Input: part model. Units: mm. Frame: model coordinates. Face numbers are marked on the shaded views. Give positions to 0.01 mm unless a question says otherwise; leave off trailing zeros. Order: outer loops, then holes, each group sorted by start corner. A loop starts at its lowest first (then second) coordinate and runs counter-clockwise, first axis right, second up.
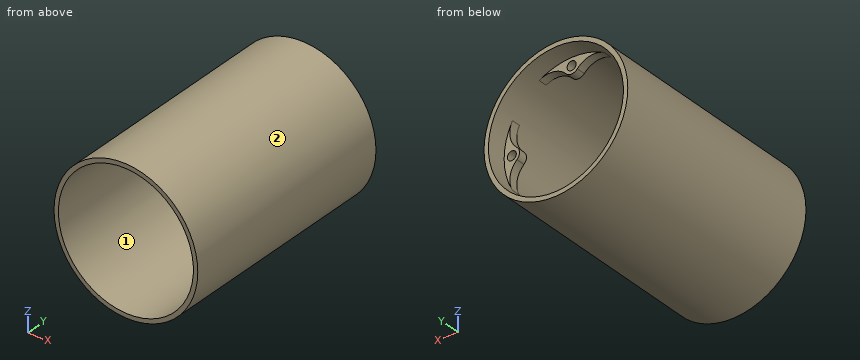
```python
from build123d import *

# Parameters (mm, degrees)
SKETCH1_R           = 32.75
SKETCH1_R_2         = 30.75
BOSS_EXTRUDE1_DEPTH = 102
SKETCH3_R           = 2.05
BOSS_EXTRUDE2_DEPTH = 4
FILLET1_R           = 10


with BuildPart() as part:
    # Sketch1 → Boss-Extrude1 (new body)
    with BuildSketch(Plane(origin=(0, 0, 0), x_dir=(1, 0, 0), z_dir=(0, 1, 0))):
        with Locations(Location((0, 0, 0), (0, 0, 270))):
            Circle(SKETCH1_R)
        with Locations(Location((0, 0, 0), (0, 0, 270))):
            Circle(SKETCH1_R_2, mode=Mode.SUBTRACT)
    extrude(amount=BOSS_EXTRUDE1_DEPTH)

    # Sketch3 → Boss-Extrude2 (add)
    # profile 1 of 4: a face of its own
    with BuildSketch(Plane(origin=(0, 93, 0), x_dir=(1, 0, 0), z_dir=(0, 1, 0))):
        with BuildLine():
            Line((-3.5, 27.25), (-3.5, 30.801785663))
            ThreePointArc((-3.5, 30.801785663), (0, 31), (3.5, 30.801785663))
            Line((3.5, 30.801785663), (3.5, 27.25))
            ThreePointArc((3.5, 27.25), (0, 23.75), (-3.5, 27.25))
        make_face()
        with Locations(Location((0, 27.25, 0), (0, 0, 270))):
            Circle(SKETCH3_R, mode=Mode.SUBTRACT)
    # profile 2 of 4: a face of its own
    with BuildSketch(Plane(origin=(0, 93, 0), x_dir=(1, 0, 0), z_dir=(0, 1, 0))):
        with BuildLine():
            Line((27.25, -3.5), (30.801785663, -3.5))
            ThreePointArc((30.801785663, -3.5), (31, 0), (30.801785663, 3.5))
            Line((30.801785663, 3.5), (27.25, 3.5))
            ThreePointArc((27.25, 3.5), (23.75, 0), (27.25, -3.5))
        make_face()
        with Locations(Location((27.25, 0, 0), (0, 0, 270))):
            Circle(SKETCH3_R, mode=Mode.SUBTRACT)
    # profile 3 of 4: a face of its own
    with BuildSketch(Plane(origin=(0, 93, 0), x_dir=(1, 0, 0), z_dir=(0, 1, 0))):
        with BuildLine():
            Line((-3.5, -27.25), (-3.5, -30.801785663))
            ThreePointArc((-3.5, -30.801785663), (0, -31), (3.5, -30.801785663))
            Line((3.5, -30.801785663), (3.5, -27.25))
            ThreePointArc((3.5, -27.25), (0, -23.75), (-3.5, -27.25))
        make_face()
        with Locations(Location((0, -27.25, 0), (0, 0, 270))):
            Circle(SKETCH3_R, mode=Mode.SUBTRACT)
    # profile 4 of 4: a face of its own
    with BuildSketch(Plane(origin=(0, 93, 0), x_dir=(1, 0, 0), z_dir=(0, 1, 0))):
        with BuildLine():
            Line((-27.25, 3.5), (-30.801785663, 3.5))
            ThreePointArc((-30.801785663, 3.5), (-31, 0), (-30.801785663, -3.5))
            Line((-30.801785663, -3.5), (-27.25, -3.5))
            ThreePointArc((-27.25, -3.5), (-23.75, 0), (-27.25, 3.5))
        make_face()
        with Locations(Location((-27.25, 0, 0), (0, 0, 270))):
            Circle(SKETCH3_R, mode=Mode.SUBTRACT)
    extrude(amount=-BOSS_EXTRUDE2_DEPTH)

    # Fillet1
    # the kernel refuses this fillet: 10 mm, written as the material it adds along each edge
    with BuildSketch(Plane(origin=(30.550163666, 93, 3.5), x_dir=(-0.30360135292633833, 0, 0.9527991490872024), z_dir=(0, -1, 0)), Plane(origin=(-3.5, 93, 30.550163666), x_dir=(-0.9527991490872014, 0, -0.30360135292634133), z_dir=(0, -1, 0)), Plane(origin=(-30.550163666, 93, -3.5), x_dir=(0.3036013529263449, 0, -0.9527991490872003), z_dir=(0, -1, 0)), Plane(origin=(3.5, 93, -30.550163666), x_dir=(0.9527991490872035, 0, 0.30360135292633456), z_dir=(0, -1, 0))) as fillet1_piece_1:
        with BuildLine():
            CenterArc((9.948751576, 9.811634042), FILLET1_R, 204.529281699, 76.609121242)
            Line((0.851259395, 5.660051691), (-0.058489823, 5.244893456))
            ThreePointArc((-0.058489823, 5.244893456), (0.049135005, 3.447994485), (-0.952799149, 0.303601353))
            Line((-0.952799149, 0.303601353), (-0.193179642, -0.981163404))
            ThreePointArc((-0.193179642, -0.981163404), (5.940273999, -1.57922532), (12.073727641, -0.981163404))
            Line((12.073727641, -0.981163404), (11.880547998, 0))
        make_face()
    extrude(amount=4)
    with BuildSketch(Plane(origin=(30.550163666, 93, -3.5), x_dir=(-0.3036013529263308, 0, -0.9527991490872049), z_dir=(0, -1, 0)), Plane(origin=(3.5, 93, 30.550163666), x_dir=(0.9527991490872056, 0, -0.3036013529263281), z_dir=(0, -1, 0)), Plane(origin=(-30.550163666, 93, 3.5), x_dir=(0.30360135292632445, 0, 0.9527991490872069), z_dir=(0, -1, 0)), Plane(origin=(-3.5, 93, -30.550163666), x_dir=(-0.9527991490872035, 0, 0.30360135292633467), z_dir=(0, -1, 0))) as fillet1_piece_2:
        with BuildLine():
            CenterArc((9.948751576, -9.811634042), FILLET1_R, 78.861597059, 76.609121242)
            Line((0.851259395, -5.660051691), (-0.058489823, -5.244893456))
            ThreePointArc((-0.058489823, -5.244893456), (0.049135005, -3.447994485), (-0.952799149, -0.303601353))
            Line((-0.952799149, -0.303601353), (-0.193179642, 0.981163404))
            ThreePointArc((-0.193179642, 0.981163404), (5.940273999, 1.57922532), (12.073727641, 0.981163404))
            Line((12.073727641, 0.981163404), (11.880547998, 0))
        make_face()
    extrude(amount=4)


solid = part.part
```
1) First-contact query: P1, Ø5.5, axis at x = -7, z = -27, coming from the -Y side; P2, Ø3.5, axis at x = 4.5, z = -27, coming from the +Y side; P3, Ø1, axis at y = 21, z = -11, coming from the +X side; P4, Ø12, axis at x = 25, z = 11, coming from the -Y side. Flat tips, straight axial feed; report the tip coordinate or a pass-through.
2) Line query: probe 1 along X at (y, z) = (91.15, 27.25); probe 2 along Z at (x, y) = (-27, 91); probe 3 along X at (y, z) = (21, -12). Output: solid intervals per line, ascending.
3) Cut plane B-B (z = -7.5). Return the cut outline in (x, y), then the cut area to 3 significant figures.
4) Cut plane A-A (x = 0). Return the cut outline in (y, z), then the cut area to 3 significant figures.
5) Pull-direction query (Z, two-part tool) for the marked faces 1 and 2; classes: pulls with the +Z half, pulls with the -Z half, needs draft (parallel to the pull), parting line crosses it, or undercut.
6) Cut plane D-D (y = 16). Return the cut outline in (x, z).
7) Cut plane C-C (x = 21.5). Return the cut outline in (y, z).
Geometry says:
1. P1: stops at y = 89
1. P2: stops at y = 93
1. P3: stops at x = 31.02
1. P4: stops at y = 0
2. probe 1: x = -18.17 to -14.21, -5.79 to -2.05, 2.05 to 5.79, 14.21 to 18.17
2. probe 2: z = -18.54 to -14.72, -5.29 to -2.03, 2.03 to 5.29, 14.72 to 18.54
2. probe 3: x = -30.47 to -28.31, 28.31 to 30.47
3. outline: (-31.88, 0) - (-29.82, 0) - (-29.82, 89) - (-27.86, 89) - (-27.86, 93) - (-29.82, 93) - (-29.82, 102) - (-31.88, 102) - close; (27.86, 89) - (29.82, 89) - (29.82, 0) - (31.88, 0) - (31.88, 102) - (29.82, 102) - (29.82, 93) - (27.86, 93) - close
3. area: 436 mm2
4. outline: (0, -32.75) - (102, -32.75) - (102, -30.75) - (93, -30.75) - (93, -29.3) - (89, -29.3) - (89, -30.75) - (0, -30.75) - close; (0, 30.75) - (89, 30.75) - (89, 29.3) - (93, 29.3) - (93, 30.75) - (102, 30.75) - (102, 32.75) - (0, 32.75) - close; (89, -25.2) - (93, -25.2) - (93, -23.75) - (89, -23.75) - close; (89, 23.75) - (93, 23.75) - (93, 25.2) - (89, 25.2) - close
4. area: 431 mm2
5. face 1: undercut
5. face 2: parting line crosses it
6. outline: circle Ø65.5 at (0, 0); hole circle Ø61.5 at (0, 0)
7. outline: (0, -24.7) - (102, -24.7) - (102, -21.98) - (0, -21.98) - close; (0, 21.98) - (102, 21.98) - (102, 24.7) - (0, 24.7) - close
